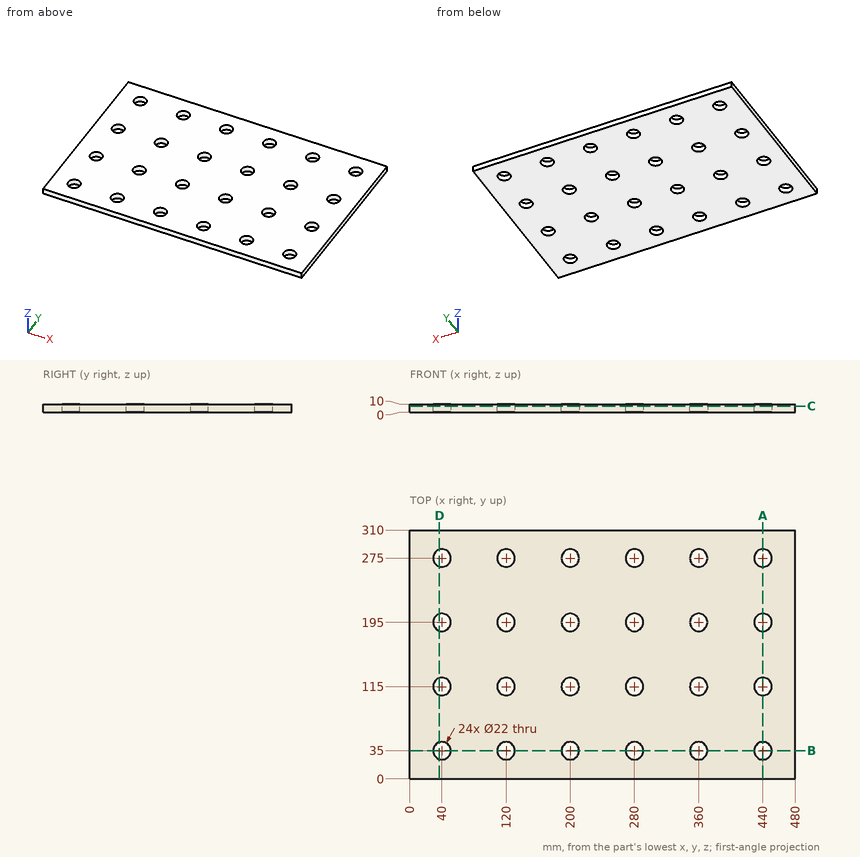
Answer from the drawing. Dimensions are ordinates in mm from the lowest x, y and z of the part. Round coordinates to 2 decimals unless told otherwise and drop trailing zeros. Write each loop counter-clockwise with the first axis right and the second up, starting at its lowest first coordinate (ties: lowest second). Pieces come first, ordered by that corner, then holes. Notation, with made-up numbers: M 24.5,77 L 53.5,77 A19 cw 53.5,100 Z; hole C -15,29.25 d9. An arc over 180 degrees is marked long. Write each question's results on one line, items separated by ' | '. Start each with the question number.
Item 1: A cutting plane is placed at D-D on x = 37. Write down the section's boundary in (y, z), and give its area (3 significant figures).
Item 2: Straight lines are drawn through the part: L1, parallel to Y at x = 120, z = 3; L2, parallel to Y at x = 43, z = 5.25. For each, find the intervals that lie inside material, in ascending order. Write a range as [from, to].
Item 3: A cutting plane is placed at A-A on x = 440. Write down the section's boundary in (y, z), and give its area (3 significant figures).
Item 4: A flat-ended cylindrical pin translates along its axis: pin 1 Ø3 at (y, z) = (45, 8) entering from -X. Find the tip coordinate at first contact, or state that the pin passes through.
Item 5: A cutting plane is placed at B-B on y = 35. Write down the section's boundary in (x, z).
Item 6: A cutting plane is placed at C-C on z = 7.25. State how many separate pieces and enclosed holes the cut face has, and give its area (3 significant figures).
Check sheet entries:
1) outline: M 0,0 L 24.42,0 L 24.42,10 L 0,10 Z; M 45.58,0 L 104.42,0 L 104.42,10 L 45.58,10 Z; M 125.58,0 L 184.42,0 L 184.42,10 L 125.58,10 Z; M 205.58,0 L 264.42,0 L 264.42,10 L 205.58,10 Z; M 285.58,0 L 310,0 L 310,10 L 285.58,10 Z | area: 2,250 mm²
2) L1: [0, 24], [46, 104], [126, 184], [206, 264], [286, 310] | L2: [0, 24.42], [45.58, 104.42], [125.58, 184.42], [205.58, 264.42], [285.58, 310]
3) outline: M 0,0 L 24,0 L 24,10 L 0,10 Z; M 46,0 L 104,0 L 104,10 L 46,10 Z; M 126,0 L 184,0 L 184,10 L 126,10 Z; M 206,0 L 264,0 L 264,10 L 206,10 Z; M 286,0 L 310,0 L 310,10 L 286,10 Z | area: 2,220 mm²
4) pin 1: x = 0
5) outline: M 0,0 L 29,0 L 29,10 L 0,10 Z; M 51,0 L 109,0 L 109,10 L 51,10 Z; M 131,0 L 189,0 L 189,10 L 131,10 Z; M 211,0 L 269,0 L 269,10 L 211,10 Z; M 291,0 L 349,0 L 349,10 L 291,10 Z; M 371,0 L 429,0 L 429,10 L 371,10 Z; M 451,0 L 480,0 L 480,10 L 451,10 Z
6) separate pieces: 1 | enclosed holes: 24 | area: 140,000 mm²
